Input: part model. Units: mm. Frame: model coordinates. A direction names the side the tool comes from. Give positions to 0.01 mm unless a question says otherwise; leave off trailing zeros. Loops run counter-clockwise (first coordinate to the right, second up) from the corner with the lowest first, then second, coordinate; pieces in that order, holes last. Notation, with made-up numbers: (35.25, -34.75) - (56.25, -34.75) arc R9 cw to (56.25, -26.75) - close; hole circle Ø4 at (-7.5, 36.25). An arc over 180 degrees is marked (long way). One line per item, written item: value.
from build123d import *

# Parameters (mm, degrees)
SKETCH1_W           = 54
SKETCH1_H           = 34
SKETCH1_R           = 1
BOSS_EXTRUDE1_DEPTH = 5
FILLET2_R           = 3
SKETCH2_R           = 2.5
CUT_EXTRUDE1_DEPTH  = 3


with BuildPart() as part:
    # Sketch1 → Boss-Extrude1 (new body)
    with BuildSketch(Plane.XY):
        with Locations((27, -17)):
            Rectangle(SKETCH1_W, SKETCH1_H)
        with Locations((5, -5)):
            Circle(SKETCH1_R, mode=Mode.SUBTRACT)
        with Locations((49, -5)):
            Circle(SKETCH1_R, mode=Mode.SUBTRACT)
        with Locations((49, -29)):
            Circle(SKETCH1_R, mode=Mode.SUBTRACT)
        with Locations((5, -29)):
            Circle(SKETCH1_R, mode=Mode.SUBTRACT)
    extrude(amount=BOSS_EXTRUDE1_DEPTH)

    # Fillet2
    fillet2_edges = [part.edges().sort_by_distance(p)[0] for p in [
        (54, -17, 5),
        (27, 0, 5),
        (0, -17, 5),
        (0, 0, 2.5),
        (54, 0, 2.5),
        (54, -34, 2.5),
        (0, -34, 2.5),
        (27, -34, 5),
    ]]
    fillet(fillet2_edges, radius=FILLET2_R)

    # Sketch2 → Cut-Extrude1 (cut)
    with BuildSketch(Plane.XY.offset(5)):
        with Locations((5, -5)):
            Circle(SKETCH2_R)
        with Locations((5, -29)):
            Circle(SKETCH2_R)
        with Locations((49, -29)):
            Circle(SKETCH2_R)
        with Locations((49, -5)):
            Circle(SKETCH2_R)
    extrude(amount=-CUT_EXTRUDE1_DEPTH, mode=Mode.SUBTRACT)


solid = part.part
Item 1: Section C-C, the plane y = -5. Output: boundary loops of the cut face in (x, z), and give its area (3 significant figures).
Verdict:
outline: (0, 0) - (4, 0) - (4, 2) - (2.5, 2) - (2.5, 4.96) arc R3 ccw to (0, 2) - close; (6, 0) - (48, 0) - (48, 2) - (46.5, 2) - (46.5, 5) - (7.5, 5) - (7.5, 2) - (6, 2) - close; (50, 0) - (54, 0) - (54, 2) arc R3 ccw to (51.5, 4.96) - (51.5, 2) - (50, 2) - close
area: 228 mm^2
Item 2: Section A-A, the plane z = 3.8. Output: boundary loops of the cut face in (x, y), and give its area (3 significant figures).
Verdict:
outline: (0.6, -31) arc R2.4 ccw to (3, -33.4) - (51, -33.4) arc R2.4 ccw to (53.4, -31) - (53.4, -3) arc R2.4 ccw to (51, -0.6) - (3, -0.6) arc R2.4 ccw to (0.6, -3) - close; hole circle Ø5 at (5, -29); hole circle Ø5 at (5, -5); hole circle Ø5 at (49, -29); hole circle Ø5 at (49, -5)
area: 1,650 mm^2
Item 3: Material intervals for L1, parallel to Y at x = 49, z = 0.6; L2, parallel to X at y = -29, z = 3.25; L3, parallel to Y at x = 49, z = 2.85, sorted ascending.
Verdict:
L1: y = -34 to -30, -28 to -6, -4 to 0
L2: x = 0.27 to 2.5, 7.5 to 46.5, 51.5 to 53.73
L3: y = -33.88 to -31.5, -26.5 to -7.5, -2.5 to -0.12
Item 4: Pin query (flat end, axial travel): P1, Ø2.5, axis at x = 49, y = -4.5, coming from the +Z side; P2, Ø1.8, axis at x = 49, y = -5, coming from the -Z side; P3, Ø1.5, axis at y = -8.5, z = 4, coming from the +X side; P4, Ø1, axis at y = -27.5, z = 3.5, coming from the -X side. Return the tip coordinate at first contact, or that it passes through.
Verdict:
P1: stops at z = 2
P2: passes through
P3: stops at x = 53.73
P4: stops at x = 0.17
Item 5: Section B-B, the plane x = 5. Output: boundary loops of the cut face in (y, z).
Verdict:
outline: (-34, 0) - (-30, 0) - (-30, 2) - (-31.5, 2) - (-31.5, 4.96) arc R3 ccw to (-34, 2) - close; (-28, 0) - (-6, 0) - (-6, 2) - (-7.5, 2) - (-7.5, 5) - (-26.5, 5) - (-26.5, 2) - (-28, 2) - close; (-4, 0) - (0, 0) - (0, 2) arc R3 ccw to (-2.5, 4.96) - (-2.5, 2) - (-4, 2) - close
Item 6: Access query for faces 1 (the face through (0, -17, 1)), 2 (the face through (7.385, -4.249, 3.521)). Directions: +Z, -Z, +X, -X, +Y, -Y. A direction counts if a zero-diameter tool reaches every point of the face in a straight line with its end or side. Return the directions, or none.
Verdict:
face 1: +Z, -Z, -X, +Y, -Y
face 2: +Z
Item 7: Draft query along X for faces 3 (the face through (49.54, -28.16, 0.99)), 4 (the face through (54, -17, 1)), 5 (the face through (27, -34, 1)). Return one class per face: pulls with the +X half, pulls with the -X half, needs draft (parallel to the pull), parting line crosses it, or undercut.
Verdict:
face 3: undercut
face 4: pulls with the +X half
face 5: needs draft
Item 8: Section D-D, the plane x = 17. Output: boundary loops of the cut face in (y, z).
Verdict:
outline: (-34, 0) - (0, 0) - (0, 2) arc R3 ccw to (-3, 5) - (-31, 5) arc R3 ccw to (-34, 2) - close
